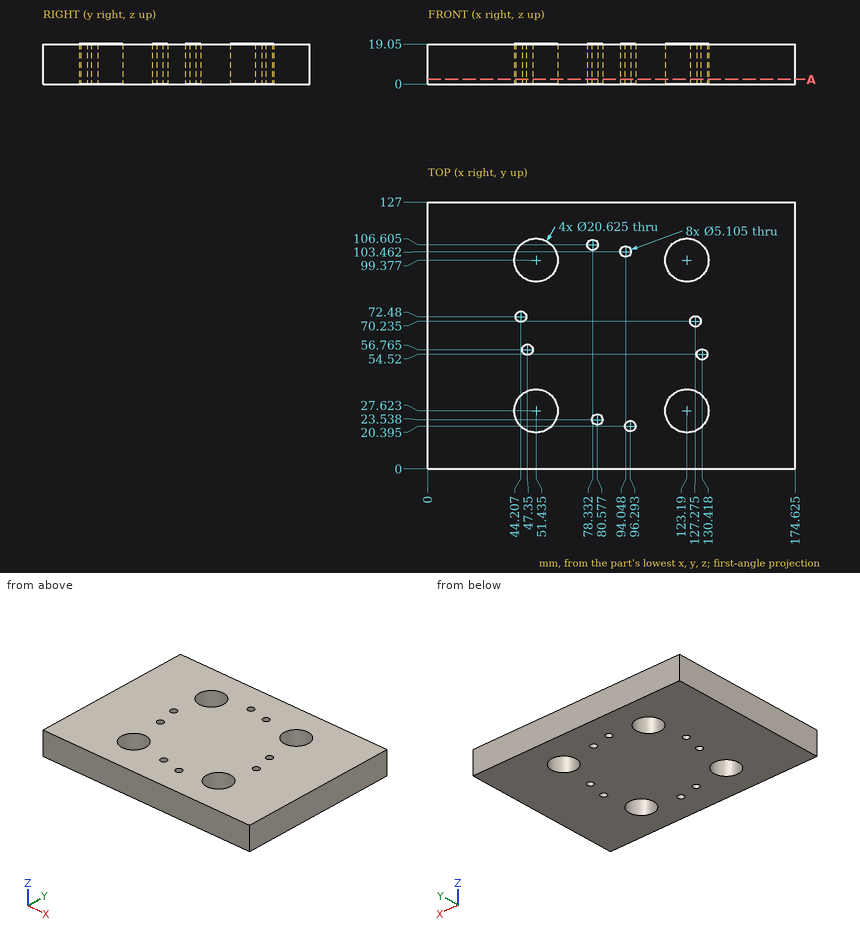
Design review of the part shown in the three views and the two pictorial views. Dimensions are in mm from the part's minimum x, y and z. Give positions to 0.01 mm unless a question says otherwise; leave off trailing zeros. Answer in a Markdown table with one row per item.
1) For L1, parallel to X at y = 28, z = 10 (1 decimal); L2, parallel to X at y = 30, z = 8.5 (1 decimal); L3, parallel to X at y = 24, z = 2.25 (1 decimal), list the stretches that pass through material, from the lowest coordinate up. Write a range as [from, to].
Worked answers:
| item | result |
|---|---|
| L1 | [0, 41.1], [61.7, 112.9], [133.5, 174.6] |
| L2 | [0, 41.4], [61.5, 113.2], [133.2, 174.6] |
| L3 | [0, 41.8], [61.1, 78.1], [83.1, 113.5], [132.8, 174.6] |
2) Clearance check with flat-ended pins moving along their axes: P1, Ø4.5, axis at x = 96.29, y = 20.39, coming from the -Z side; P2, Ø6, axis at x = 108.5, y = 64.5, coming from the -Z side. State where each tip first meets the part, or that it passes through.
Worked answers:
| item | result |
|---|---|
| P1 | through |
| P2 | z = 0 |
3) Add section A-A on z = 2.25. Count the separate pieces of the cut face and the enclosed holes in it, plus the area to 3 significant figures.
Worked answers:
| item | result |
|---|---|
| separate pieces | 1 |
| enclosed holes | 12 |
| area | 20,700 mm² |
